from build123d import *

# Parameters (mm, degrees)
F0_R      = 4.25
F1_DEPTH  = 33
F2_DEPTH  = 6
F3_R      = 7.5
F3_R_2    = 4.25
F4_DEPTH  = 2.5
F6_DEPTH  = 18
F7_R      = 0.5
F8_R      = 1
F10_R     = 1.5
F11_DEPTH = 40
F12_DEPTH = 25


with BuildPart() as f1:
    # F0 (on Front) → F1 (new body)
    with BuildSketch(Plane.XZ):
        Circle(F0_R)
        Polygon((-1.375, 2.38157), (2.75, 0), (-1.375, -2.38157), align=None, mode=Mode.SUBTRACT)
        Polygon((-1.375, -2.38157), (2.75, 0), (-1.375, 2.38157), align=None)
    extrude(amount=F1_DEPTH)

    # F0 (on Front) → F2 (cut)
    with BuildSketch(Plane.XZ):
        Polygon((-1.375, -2.38157), (2.75, 0), (-1.375, 2.38157), align=None)
    extrude(amount=F2_DEPTH, mode=Mode.SUBTRACT)

    # F3 (on face) → F4 (join)
    with BuildSketch(Plane.XZ.offset(33)):
        Circle(F3_R)
        Circle(F3_R_2, mode=Mode.SUBTRACT)
        Circle(F3_R_2)
    extrude(amount=F4_DEPTH)

    # F5 (on face) → F6 (join)
    with BuildSketch(Plane.XZ.offset(35.5)):
        Polygon((0.076423, -4.499351), (3.934764, -2.183492), (3.858341, 2.315859), (-0.076423, 4.499351), (-3.934764, 2.183492), (-3.858341, -2.315859), align=None)
    extrude(amount=F6_DEPTH)

    # F7
    f7_edges = [f1.edges().sort_by_distance(p)[0] for p in [
        (2.005593, -53.5, -3.341421),
        (-1.890959, -53.5, -3.407605),
        (-3.896552, -53.5, -0.066184),
        (-2.005593, -53.5, 3.341421),
        (1.890959, -53.5, 3.407605),
        (3.896552, -53.5, 0.066184),
    ]]
    fillet(f7_edges, radius=F7_R)

    # F8
    f8_edges = [f1.edges().sort_by_distance(p)[0] for p in [
        (-7.5, -35.5, 0),
        (-7.5, -33, 0),
    ]]
    fillet(f8_edges, radius=F8_R)

    # F10 (on offset) → F11 (cut)
    with BuildSketch(Plane.XY.offset(25)):
        with Locations((0, -18)):
            Circle(F10_R)
    extrude(amount=-F11_DEPTH, mode=Mode.SUBTRACT)

    # F0 (on Front) → F12 (join)
    with BuildSketch(Plane.XZ):
        Polygon((-1.375, -2.38157), (2.75, 0), (-1.375, 2.38157), align=None)
    extrude(amount=F12_DEPTH)


solid = f1.part
Geometry check sheet. Reference: the model listing, model coordinates, mm. A direction names the side the tool comes from. Coordinates: 2 decimals unless noted, no trailing zeros. Order: outer loops, then holes, each group sorted by start corner. A loop starts at its lowest first (then second) coordinate and runs counter-clockwise, first axis right, second up. Notation, with made-up numbers: (66, 71.25) -> (98, 71.25) arc R18 cw to (98, 91.25) -> close; hole circle Ø7 at (-20.75, -17). An arc over 180 degrees is marked (long way). Use a Markdown table: item, result. Add a question column.
1. Go/stop test with flat-tipped pins: pin 1 Ø1.5 at (y, z) = (-7.5, 0.5) entering from -X; pin 2 Ø4 at (x, y) = (2.5, -15.5) entering from +Z; pin 3 Ø4 at (y, z) = (-21, 5) entering from -X. Record where each tip stops, or that it passes through.
2. Mould release check, pull along Y, two halves, no side actions. Record for faces 4 (the face through (0, 0, 0)), 5 (the face through (1.979, -44.128, -3.358)), 6 (the face through (0.08, -17.98, 1.54)): pulls with the +Y half, pulls with the -Y half, needs draft (parallel to the pull), parting line crosses it, or undercut.
3. Set-up check for faces 1 (the face through (-1.979, -44.128, 3.358)), 2 (the face through (1.92, -44.13, 3.39)), 3 (the face through (2.285, -16.269, 3.584)): record each of +Z, -Z, +X, -X, +Y, -Y from which the full face is reachable in a straight line by a thin tool's end or side.
4. Cross-section at B-B (y = -42). Enter the section's corners in (x, z).
5. Material ranges on L1, parallel to Y at x = 0, z = -2.5; L2, parallel to Z at x = -2.5, y = -22; L3, parallel to Y at x = -5, z = -3.75, recorded low to high.
Filled sheet:
| question | item | result |
|---|---|---|
| 1 | pin 1 | x = -4.25 |
| 1 | pin 2 | z = 4.22 |
| 1 | pin 3 | x = -3.01 |
| 2 | face 4 | pulls with the +Y half |
| 2 | face 5 | needs draft |
| 2 | face 6 | undercut |
| 3 | face 1 | +Z, -X, -Y |
| 3 | face 2 | +Z, +X, -Y |
| 3 | face 3 | +Y |
| 4 | outline | (-3.93, 2.18) -> (-3.86, -2.32) -> (0.08, -4.5) -> (3.93, -2.18) -> (3.86, 2.32) -> (-0.08, 4.5) -> close |
| 5 | L1 | -53.5 to -19.5, -16.5 to 0 |
| 5 | L2 | -3.44 to 3.44 |
| 5 | L3 | -35.5 to -33 |
